Model file for the job. Use its own axes, mm. A direction names the side the tool comes from. Round coordinates to 2 decimals unless told otherwise and drop trailing zeros. Write each loop counter-clockwise with the first axis right and the second up, starting at its lowest first coordinate (ties: lowest second). Pieces come first, ordered by that corner, then holes. Notation, with made-up numbers: (-18.75, 36.5) - (8.25, 36.5) arc R16 ccw to (8.25, 53.5) - close; hole circle Ø1 at (-24, -30.5). An arc over 180 degrees is marked (long way). One line per item, written item: value.
from build123d import *

# Parameters (mm, degrees)
F1_DEPTH = 102
F2_DEPTH = 60


with BuildPart() as f1:
    # F0 (on Right) → F1 (new body, symmetric)
    with BuildSketch(Plane.YZ):
        Polygon((9, 23), (0, 0), (204, 0), (204, 23), (113, 23), (61, 23), align=None)
    extrude(amount=F1_DEPTH, both=True)

    # F0 (on Right) → F2 (join, symmetric)
    with BuildSketch(Plane.YZ):
        Polygon((61, 85), (61, 23), (113, 23), (113, 35), (73, 35), (73, 85), (69, 85), (69, 81), (65, 81), (65, 85), align=None)
    extrude(amount=F2_DEPTH, both=True)


solid = f1.part
1. Band-saw the part on C-C on z = 70.5. Write the cut outline in (x, y).
Report:
outline: (-60, 61) - (60, 61) - (60, 73) - (-60, 73) - close
2. Band-saw the part on A-A on x = -42.5. Write the cut outline in (y, z), plus the area to 3 significant figures.
Report:
outline: (0, 0) - (204, 0) - (204, 23) - (113, 23) - (113, 35) - (73, 35) - (73, 85) - (69, 85) - (69, 81) - (65, 81) - (65, 85) - (61, 85) - (61, 23) - (9, 23) - close
area: 5,800 mm²
3. Drop flat-ended pins along their axis: pin 1 (1.2 mm diameter, centred on x = 2.5, z = 83.5, fed in from -Y); pin 2 (2 mm diameter, centred on x = -14.5, z = 82.5, fed in from +Y); pin 3 (1 mm diameter, centred on x = 74, y = 103.5, fed in from +Z). Give the stop position or say it passes through.
Report:
pin 1: y = 61
pin 2: y = 73
pin 3: z = 23
4. Tool access for faces 1 (the face through (-60, 69, 41)), 2 (the face through (1, 61, 54)), 3 (the face through (1, 73, 60)): list every direction of +Z, -Z, +X, -X, +Y, -Y with a clear straight run to the whole face (end or side of a thin tool).
Report:
face 1: +Z, -X, +Y, -Y
face 2: +Z, +X, -X, -Y
face 3: +Z, +X, -X, +Y
5. Band-saw the part on B-B on y = 34. Write the cut outline in (x, z), plus the area to 3 significant figures.
Report:
outline: (-102, 0) - (102, 0) - (102, 23) - (-102, 23) - close
area: 4,690 mm²
6. Wall check: probe 1 along Y at (x, z) = (-47, 74); probe 2 along Z at (x, y) = (33, 191.5); probe 3 along Z at (x, y) = (31, 110). Give the ranges that are in metal, low to high. Write a range as [from, to].
Report:
probe 1: [61, 73]
probe 2: [0, 23]
probe 3: [0, 35]
